Source: CAD feature listing. Evaluate the final solid. Frame: model axes, mm. A direction names the side the tool comes from. Coordinates: 2 decimals unless noted, no trailing zeros. Loops run counter-clockwise (first coordinate to the right, second up) from the corner with the lowest first, then second, coordinate; pieces in that order, holes last. Notation, with made-up numbers: M 34,25.25 L 50,25.25 A16 ccw 50,45.25 Z; hole C -3,-29.75 d8. An arc over 180 degrees is marked long. One line per question, with ' | ' between items. Start each with the question number.
1. Section query B-B, the plane z = 46.5. State how many separate pieces and enclosed holes the cut face has, and give its area (3 significant figures).
2. Section query D-D, the plane z = 21. Output: boundary loops of the cut face in (x, y).
3. Section query A-A, the plane y = 31. Output: boundary loops of the cut face in (x, z), and give its area (3 significant figures).
4. Pin query (flat end, axial travel): P1, Ø4, axis at y = 15, z = -20.5, coming from the -X side; P2, Ø3, axis at x = 16.5, z = 6.5, coming from the -Y side; P3, Ø1.8, axis at y = 33.5, z = 50.5, coming from the +X side. Return the tip coordinate at first contact, or that it passes through.
5. Ray query, probe 1 along X at (y, z) = (23, 43.5); probe 2 along X at (y, z) = (23, 47); probe 3 along X at (y, z) = (10.05, 47.25). Return the intervals inside material, ascending.
6. Access query for faces 4 (the flat face through (0, 34.3, 49)), 5 (the flat face through (0, 15, -53.65)), 6 (the flat face through (0, 1.3, 40)), 7 (the flat face through (0, 7.9, -11)), 8 (the flat face through (-11, 28.1, -47)). Directions: +Z, -Z, +X, -X, +Y, -Y. A direction counts if a zero-diameter tool reaches every point of the face in a straight line with its end or side. Return the directions, or none.
7. Mould query, pull axis Z, two halves, no side actions, for faces 1 (the flat face through (0, 7, 43.65)), 2 (the cylindrical face through (19.86, 18.77, 20.76)), 3 (the cylindrical face through (17.712, 12.587, -49.785)). Classes: pulls with the +Z half, pulls with the -Z half, needs draft (parallel to the pull), parting line crosses it, or undercut.
```python
from build123d import *

# Parameters (mm, degrees)
BOSS_EXTRUDE1_DEPTH     = 33.8
CUT_EXTRUDE1_DEPTH      = 25
CUT_EXTRUDE1_DEPTH_BACK = 25
SKETCH3_W               = 42
SKETCH3_H               = 35
CUT_EXTRUDE2_DEPTH      = 7
SKETCH9_R               = 17.5
CUT_EXTRUDE3_DEPTH      = 28
SKETCH12_W              = 41.6
SKETCH12_H              = 2.2
CUT_EXTRUDE4_DEPTH      = 10
SKETCH13_W              = 10
SKETCH13_H              = 2.15


with BuildPart() as part:
    # Sketch1 → Boss-Extrude1 (new body)
    with BuildSketch(Plane(origin=(0, 1.3, 0), x_dir=(1, 0, 0), z_dir=(0, 1, 0))):
        with BuildLine():
            Line((-21, -22.541858429), (-21, -53.65))
            Line((-21, -53.65), (21, -53.65))
            Line((21, -53.65), (21, -22.654162541))
            ThreePointArc((21, -22.654162541), (20.938748215, -22.414370958), (20.769999986, -22.233330024))
            ThreePointArc((20.769999986, -22.233330024), (19.858228534, -20.731235829), (20.483912522, -19.089245057))
            Line((20.483912522, -19.089245057), (21.57947873, -18.064679449))
            ThreePointArc((21.57947873, -18.064679449), (22.138283161, -16.544955286), (21.250000071, -15.191154314))
            ThreePointArc((21.250000071, -15.191154314), (21.066987319, -15.008141607), (21, -14.758141571))
            Line((21, -14.758141571), (21, 53.65))
            Line((21, 53.65), (-21, 53.65))
            Line((-21, 53.65), (-21, -14.645837459))
            ThreePointArc((-21, -14.645837459), (-20.938748219, -14.885629035), (-20.77, -15.066669967))
            ThreePointArc((-20.77, -15.066669967), (-19.858228534, -16.568764162), (-20.483912522, -18.210754943))
            Line((-20.483912522, -18.210754943), (-21.57947873, -19.235320551))
            ThreePointArc((-21.57947873, -19.235320551), (-22.138283154, -20.755044775), (-21.249999964, -22.108845748))
            ThreePointArc((-21.249999964, -22.108845748), (-21.066987288, -22.291858447), (-21, -22.541858429))
        make_face()
    extrude(amount=BOSS_EXTRUDE1_DEPTH)

    # Sketch2 → Cut-Extrude1 (cut, two sides)
    with BuildSketch(Plane(origin=(0, 0, 0), x_dir=(0, 0, -1), z_dir=(1, 0, 0))) as cut_extrude1_sk:
        with BuildLine():
            Line((-26, 2.9), (-26, -8.174443219))
            Line((-26, -8.174443219), (14, -7.963716906))
            Line((14, -7.963716906), (14, 2.543524479))
            Line((14, 2.543524479), (16.45, 3.2))
            Line((16.45, 3.2), (16.45, 4.4))
            Line((16.45, 4.4), (14, 4.4))
            Line((14, 4.4), (14, 7.4))
            ThreePointArc((14, 7.4), (13.853553391, 7.753553391), (13.5, 7.9))
            Line((13.5, 7.9), (7.9, 7.9))
            ThreePointArc((7.9, 7.9), (7.546446609, 7.753553391), (7.4, 7.4))
            Line((7.4, 7.4), (7.4, 4.4))
            Line((7.4, 4.4), (-19.05, 4.4))
            Line((-19.05, 4.4), (-19.05, 2.9))
            Line((-19.05, 2.9), (-26, 2.9))
        make_face()
    extrude(amount=CUT_EXTRUDE1_DEPTH, mode=Mode.SUBTRACT)
    extrude(cut_extrude1_sk.sketch, amount=-CUT_EXTRUDE1_DEPTH_BACK, mode=Mode.SUBTRACT)

    # Sketch3 → Cut-Extrude2 (cut)
    with BuildSketch(Plane(origin=(0, 35.1, 0), x_dir=(1, 0, 0), z_dir=(0, 1, 0))):
        with Locations((0, 36.15)):
            Rectangle(SKETCH3_W, SKETCH3_H)
    extrude(amount=-CUT_EXTRUDE2_DEPTH, mode=Mode.SUBTRACT)

    # Sketch4 → Cut-Revolve1 (revolve, cut)
    with BuildSketch(Plane(origin=(0, 10.05, 0), x_dir=(1, 0, 0), z_dir=(0, 1, 0))):
        Polygon((-12.15, -43.922), (-6.4275, -43.922), (-6.4275, -52.794), (-5.5715, -53.65), (-12.15, -53.65), align=None)
    revolve(axis=Axis((-12.15, 10.05, 53.65), (0, 0, -1)), mode=Mode.SUBTRACT)

    # Sketch5 → Cut-Revolve2 (revolve, cut)
    with BuildSketch(Plane(origin=(0, 10.05, 0), x_dir=(1, 0, 0), z_dir=(0, 1, 0))):
        Polygon((12.15, -43.922), (17.8725, -43.922), (17.8725, -52.794), (18.7285, -53.65), (12.15, -53.65), align=None)
    revolve(axis=Axis((12.15, 10.05, 53.65), (0, 0, -1)), mode=Mode.SUBTRACT)

    # Sketch6 → Cut-Revolve3 (revolve, cut)
    with BuildSketch(Plane(origin=(0, 23.05, 0), x_dir=(1, 0, 0), z_dir=(0, 1, 0))):
        Polygon((0, -43.922), (5.7225, -43.922), (5.7225, -52.794), (6.5785, -53.65), (0, -53.65), align=None)
    revolve(axis=Axis((0, 23.05, 53.65), (0, 0, -1)), mode=Mode.SUBTRACT)

    # Sketch7 → Cut-Revolve4 (revolve, cut)
    with BuildSketch(Plane(origin=(-15.75, 0, 0), x_dir=(0, 0, -1), z_dir=(1, 0, 0))):
        Polygon((-3.85, 27.1), (-5.471, 27.1), (-5.471, 34.721), (-5.85, 35.1), (-3.85, 35.1), align=None)
    revolve(axis=Axis((-15.75, 35.1, 3.85), (0, -1, 0)), mode=Mode.SUBTRACT)

    # Sketch8 → Cut-Revolve5 (revolve, cut)
    with BuildSketch(Plane(origin=(15.75, 0, 0), x_dir=(0, 0, -1), z_dir=(1, 0, 0))):
        Polygon((-30.35, 27.1), (-31.971, 27.1), (-31.971, 34.721), (-32.35, 35.1), (-30.35, 35.1), align=None)
    revolve(axis=Axis((15.75, 35.1, 30.35), (0, -1, 0)), mode=Mode.SUBTRACT)

    # Sketch9 → Cut-Extrude3 (cut)
    with BuildSketch(Plane(origin=(0, 35.1, 0), x_dir=(1, 0, 0), z_dir=(0, 1, 0))):
        with Locations((2.4, 35.15)):
            Circle(SKETCH9_R)
    extrude(amount=-CUT_EXTRUDE3_DEPTH, mode=Mode.SUBTRACT)

    # Sketch10 → Cut-Revolve6 (revolve, cut)
    with BuildSketch(Plane(origin=(0, 23.05, 0), x_dir=(1, 0, 0), z_dir=(0, 1, 0))):
        Polygon((-15.9, -42.65), (-14.6705, -43.359852156), (-14.6705, -53.3795), (-14.4, -53.65), (-15.9, -53.65), align=None)
    revolve(axis=Axis((-15.9, 23.05, 53.65), (0, 0, -1)), mode=Mode.SUBTRACT)

    # Sketch11 → Cut-Revolve7 (revolve, cut)
    with BuildSketch(Plane(origin=(0, 23.05, 0), x_dir=(1, 0, 0), z_dir=(0, 1, 0))):
        Polygon((16.9, -42.65), (18.1295, -43.359852156), (18.1295, -53.3795), (18.4, -53.65), (16.9, -53.65), align=None)
    revolve(axis=Axis((16.9, 23.05, 53.65), (0, 0, -1)), mode=Mode.SUBTRACT)

    # Sketch12 → Cut-Extrude4 (cut)
    with BuildSketch(Plane.XY.offset(53.65)):
        with Locations((0, 33.2)):
            Rectangle(SKETCH12_W, SKETCH12_H)
    extrude(amount=-CUT_EXTRUDE4_DEPTH, mode=Mode.SUBTRACT)

    # Sketch13 → Cut-Revolve8 (revolve, cut)
    with BuildSketch(Plane(origin=(0, 0, 0), x_dir=(0, 0, -1), z_dir=(1, 0, 0))):
        with Locations((-48.65, 8.375)):
            Rectangle(SKETCH13_W, SKETCH13_H)
    revolve(axis=Axis((0, 7.3, 43.65), (0, 0, 1)), mode=Mode.SUBTRACT)

    # Sketch14 → Cut-Revolve9 (revolve, cut)
    with BuildSketch(Plane(origin=(17.4, 0, 0), x_dir=(0, 0, -1), z_dir=(1, 0, 0))):
        Polygon((50.15, 22.1), (49.1435, 22.1), (49.1435, 27.8565), (48.9, 28.1), (50.15, 28.1), align=None)
    revolve(axis=Axis((17.4, 28.1, -50.15), (0, -1, 0)), mode=Mode.SUBTRACT)

    # Sketch15 → Cut-Revolve10 (revolve, cut)
    with BuildSketch(Plane(origin=(-16.6, 0, 0), x_dir=(0, 0, -1), z_dir=(1, 0, 0))):
        Polygon((25.15, 22.1), (24.1435, 22.1), (24.1435, 27.8565), (23.9, 28.1), (25.15, 28.1), align=None)
    revolve(axis=Axis((-16.6, 28.1, -25.15), (0, -1, 0)), mode=Mode.SUBTRACT)

    # Sketch16 → Cut-Revolve11 (revolve, cut)
    with BuildSketch(Plane(origin=(0, 13, 0), x_dir=(1, 0, 0), z_dir=(0, 1, 0))):
        Polygon((-16.4, 53.65), (-14.525, 53.65), (-15.025, 53.15), (-15.025, 44.65), (-16.4, 44.65), align=None)
    revolve(axis=Axis((-16.4, 13, -44.65), (0, 0, -1)), mode=Mode.SUBTRACT)

    # Sketch17 → Cut-Revolve12 (revolve, cut)
    with BuildSketch(Plane(origin=(0, 13, 0), x_dir=(1, 0, 0), z_dir=(0, 1, 0))):
        Polygon((16.4, 53.65), (18.275, 53.65), (17.775, 53.15), (17.775, 44.65), (16.4, 44.65), align=None)
    revolve(axis=Axis((16.4, 13, -44.65), (0, 0, -1)), mode=Mode.SUBTRACT)


solid = part.part
```
Taken from the geometry:
1) separate pieces: 1 | enclosed holes: 7 | area: 995 mm^2
2) outline: M -22.09,2.9 L 19.9,2.9 L 19.9,35.1 L -22.09,35.1 Z
3) outline: M -21.58,19.24 L -20.48,18.21 A2 cw -20.77,15.07 A0.5 ccw -21,14.65 L -21,-18.65 L -3.43,-18.65 A17.5 cw 8.23,-18.65 L 21,-18.65 L 21,14.76 A0.5 cw 21.25,15.19 A1.8 ccw 21.58,18.06 L 20.48,19.09 A2 cw 20.77,22.23 A0.5 ccw 21,22.65 L 21,53.65 L -21,53.65 L -21,22.54 A0.5 cw -21.25,22.11 A1.8 ccw Z; hole C -15.75,3.85 d3.24; hole C 15.75,30.35 d3.24 | area: 3,010 mm^2
4) P1: x = -21 | P2: y = 4.4 | P3: x = 21
5) probe 1: -21 to -17.13, -14.67 to 15.67, 18.13 to 21 | probe 2: -21 to -17.13, -14.67 to -5.72, 5.72 to 15.67, 18.13 to 21 | probe 3: -21 to -17.87, -6.43 to 6.43, 17.87 to 21
6) face 4: +Z | face 5: -Z, +X, -X, +Y, -Y | face 6: +Z, -Z, +X, -X, -Y | face 7: +X, -X, -Y | face 8: -Z, +X, -X, +Y
7) face 1: pulls with the +Z half | face 2: undercut | face 3: needs draft
